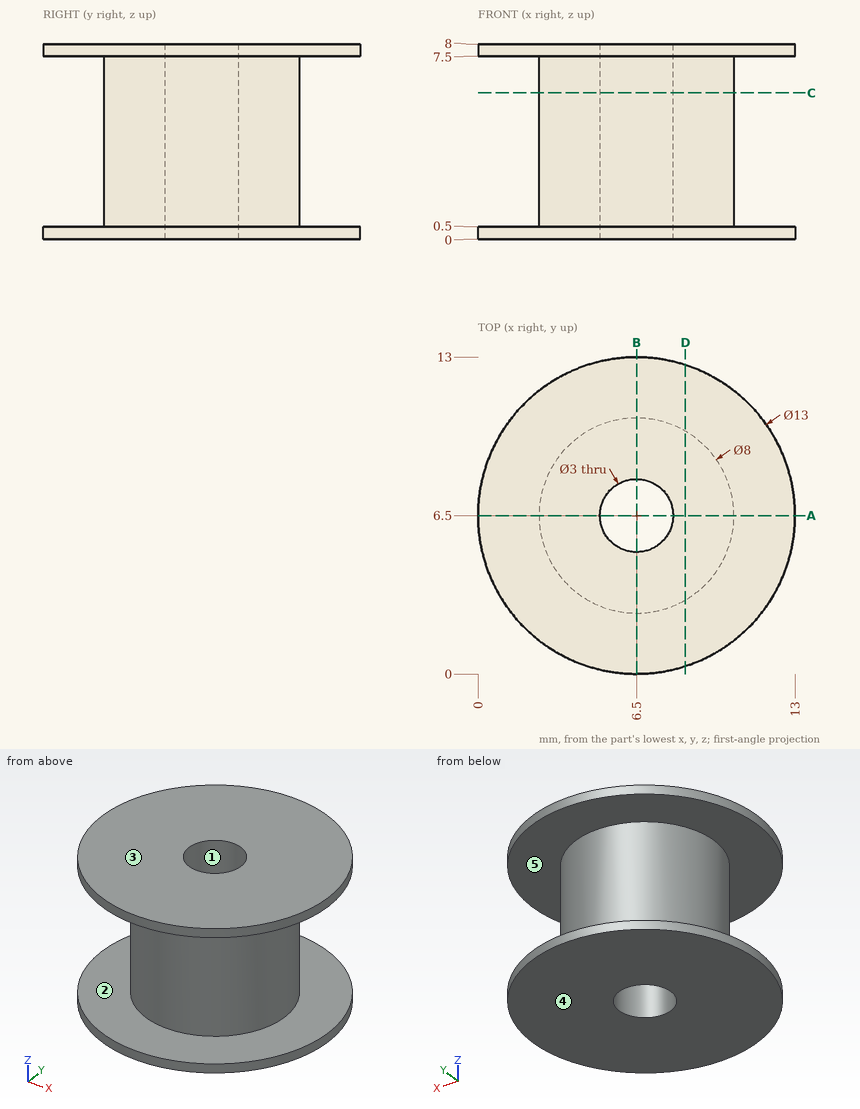
Geometry: see drawing. Coordinates: mm, zero at the bounding-box minimum. A direction names the side the tool comes from. Give positions to 0.01 mm unless a question says otherwise; leave off trailing zeros. Order: outer loops, then holes, each group sorted by start corner. A loop starts at its lowest first (then second) coordinate and runs counter-clockwise, first axis right, second up. Notation, with made-up numbers: (-12, 87) - (-4, 87) arc R34 cw to (-4, 125) - close; hole circle Ø1 at (20, 42.5). An arc over 180 degrees is marked (long way). Write each question's results on one line, items separated by ' | '.
Item 1: Draft query along Z for the marked faces 1, 2 and 3. Return one class per face: released by +Z, released by -Z, zero draft, split by the parting line, or undercut.
A:
face 1: zero draft | face 2: undercut | face 3: released by +Z
Item 2: Section C-C (z = 6). Return loops of the section in (x, y).
A:
outline: circle Ø8 at (6.5, 6.5); hole circle Ø3 at (6.5, 6.5)
Item 3: Section D-D (x = 8.5). Return loops of the section in (y, z), and give its area (3 significant figures).
A:
outline: (0.32, 0) - (12.68, 0) - (12.68, 0.5) - (9.96, 0.5) - (9.96, 7.5) - (12.68, 7.5) - (12.68, 8) - (0.32, 8) - (0.32, 7.5) - (3.04, 7.5) - (3.04, 0.5) - (0.32, 0.5) - close | area: 60.9 mm^2
Item 4: Material intervals for line 1 along Y through (x, z) = (6.5, 4); line 2 along Z through (x, y) = (3, 1.5); line 3 along X through (y, z) = (6, 3), sorted ascending.
A:
line 1: y = 2.5 to 5, 8 to 10.5 | line 2: z = 0 to 0.5, 7.5 to 8 | line 3: x = 2.53 to 5.09, 7.91 to 10.47
Item 5: Contact query for flat-ended pins moving along their axis: pin 1 Ø1 at (x, z) = (7.5, 2) entering from +Y; pin 2 Ø1.5 at (x, y) = (6, 2.5) entering from -Z. Output: stop coordinate, or through.
A:
pin 1: stops at y = 10.47 | pin 2: stops at z = 0
Item 6: Access query for the marked faces 4 and 5. Directions: +Z, -Z, +X, -X, +Y, -Y. A direction counts if a zero-diameter tool reaches every point of the face in a straight line with its end or side. Return the directions, or none.
A:
face 4: -Z, +X, -X, +Y, -Y | face 5: none
Item 7: Section A-A (y = 6.5). Return loops of the section in (x, z), and give its area (3 significant figures).
A:
outline: (0, 0) - (5, 0) - (5, 8) - (0, 8) - (0, 7.5) - (2.5, 7.5) - (2.5, 0.5) - (0, 0.5) - close; (8, 0) - (13, 0) - (13, 0.5) - (10.5, 0.5) - (10.5, 7.5) - (13, 7.5) - (13, 8) - (8, 8) - close | area: 45.0 mm^2
